Source: three-view drawing plus pictorial views. Frame: mm from the lowest corner of the part. A direction names the side the tool comes from. Give positions to 0.01 mm unless a question says otherwise; leave off trailing zeros. Loops run counter-clockwise (first coordinate to the right, second up) from the corner with the lowest first, then second, coordinate; pieces in that order, holes last. Notation, with made-up numbers: (7, 17.25) -> (11, 17.25) arc R19 cw to (11, 29.25) -> close; hole circle Ø1 at (0, 73). An arc over 180 degrees is marked (long way). One line per item, written item: value. Start each with the question number.
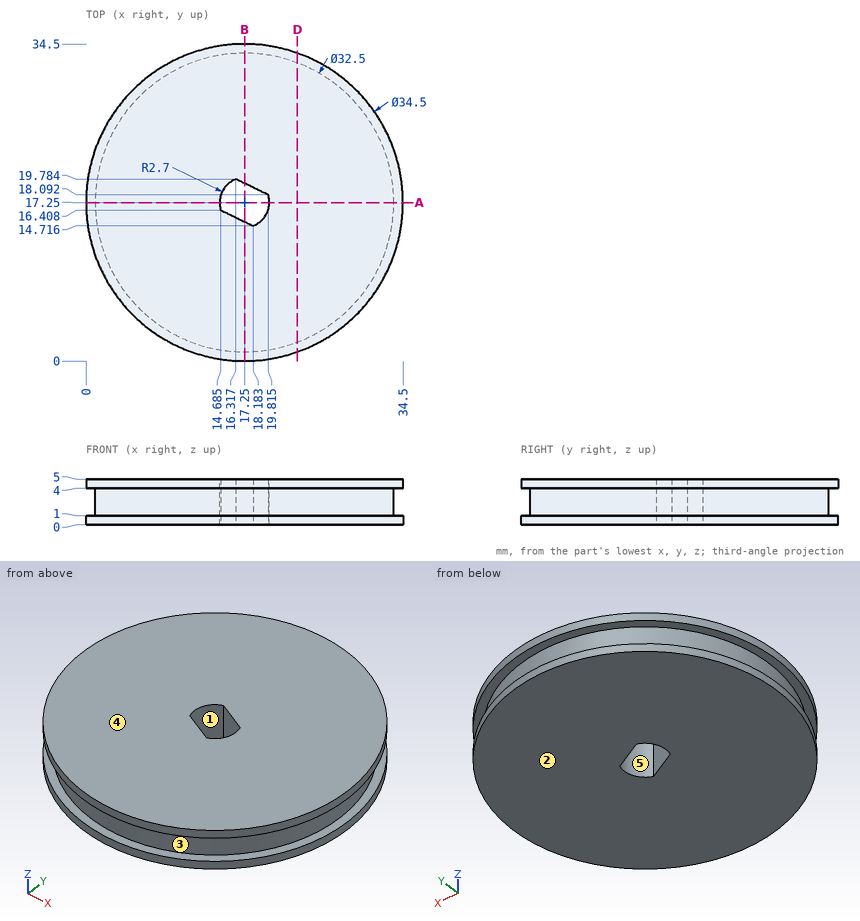
Item 1: Section A-A, the plane y = 17.25. Output: boundary loops of the cut face in (x, z).
Item 2: Ray query, line 1 along Z through (x, y) = (32, 8.5); line 2 along X through (y, z) = (15.5, 3.15) (1 decimal); line 3 along Y through (x, z) = (10.5, 0.25) (1 decimal). Return the intervals inside material, ascending. Write a range as [from, to].
Item 3: Section D-D, the plane x = 23. Output: boundary loops of the cut face in (y, z), then the cut area to 3 significant figures.
Item 4: Pin query (flat end, axial travel): pin 1 (2 mm diameter, centred on x = 8.5, z = 4, fed in from +Y); pin 2 (1.5 mm diameter, centred on y = 16, z = 2, fed in from +X); pin 3 (3 mm diameter, centred on x = 9, z = 4, fed in from +Y) (1 decimal). Return the tip coordinate at first contact, or that it passes through.
Item 5: Access query for the marked faces 1 and 2. Directions: +Z, -Z, +X, -X, +Y, -Y. A direction counts if a zero-diameter tool reaches every point of the face in a straight line with its end or side. Return the directions, or none.
Item 6: Section B-B, the plane x = 17.25. Output: boundary loops of the cut face in (y, z), then the cut area to 3 significant figures.
Item 7: Mould query, pull axis Y, two halves, no side actions, for the marked faces 3, 4 and 5. Classes: pulls with the +Y half, pulls with the -Y half, needs draft (parallel to the pull), parting line crosses it, or undercut.
Geometry check:
1. outline: (0, 0) -> (14.55, 0) -> (14.55, 5) -> (0, 5) -> (0, 4) -> (1, 4) -> (1, 1) -> (0, 1) -> close; (19.95, 0) -> (34.5, 0) -> (34.5, 1) -> (33.5, 1) -> (33.5, 4) -> (34.5, 4) -> (34.5, 5) -> (19.95, 5) -> close
2. line 1: z = [0, 1], [4, 5]
2. line 2: x = [1.1, 16.6], [19.3, 33.4]
2. line 3: y = [1.4, 33.1]
3. outline: (0.99, 0) -> (33.51, 0) -> (33.51, 1) -> (32.45, 1) -> (32.45, 4) -> (33.51, 4) -> (33.51, 5) -> (0.99, 5) -> (0.99, 4) -> (2.05, 4) -> (2.05, 1) -> (0.99, 1) -> close
3. area: 156 mm2
4. pin 1: stops at y = 32.66
4. pin 2: stops at x = 33.49
4. pin 3: stops at y = 33.1
5. face 1: +Z, -Z
5. face 2: -Z, +X, -X, +Y, -Y
6. outline: (0, 0) -> (15.17, 0) -> (15.17, 5) -> (0, 5) -> (0, 4) -> (1, 4) -> (1, 1) -> (0, 1) -> close; (19.33, 0) -> (34.5, 0) -> (34.5, 1) -> (33.5, 1) -> (33.5, 4) -> (34.5, 4) -> (34.5, 5) -> (19.33, 5) -> close
6. area: 146 mm2
7. face 3: parting line crosses it
7. face 4: needs draft
7. face 5: undercut
